Verification items for the finished model (mm, model axes). Face numbers are marked on the shaded views. A direction names the side the tool comes from. Round coordinates to 2 decimals unless told otherwise and drop trailing zeros. Order: outer loops, then holes, each group sorted by start corner. A loop starts at its lowest first (then second) coordinate and runs counter-clockwise, first axis right, second up. Notation, with made-up numbers: (5, 75.5) -> (64, 75.5) arc R13 ccw to (64, 100.5) -> close; hole circle Ø7 at (63, 32.25). An arc over 180 degrees is marked (long way). Return JSON: item names as keys, results as strings. Group by question number.
1) Scan lines: L1, parallel to Y at x = 4, z = 4.5; L2, parallel to Y at x = 76, z = 0.9; L3, parallel to X at y = 53, z = 9.5. Record each from-to range of solid material in increasing order.
2) Section check C-C on x = 18. Enter the section's corners in (y, z), plus the area to 3 significant figures.
3) Section check A-A on x = 40. Enter the section's corners in (y, z).
4) Draft check along X on the marked faces 1, 2 and 3. Enter one of: pulls with the +X half, pulls with the -X half, needs draft (parallel to the pull), parting line crosses it, or undercut.
5) Section check D-D on y = 42. Enter the section's corners in (x, z), plus the area to 3 significant figures.
6) Depth check by flat-ended pin: pin 1 (2.5 mm diameter, centred on y = 85, z = 14, fed in from -X); pin 2 (5 mm diameter, centred on y = 46.5, z = 10, fed in from -X); pin 3 (8 mm diameter, centred on x = 19, z = 9, fed in from +Y). Enter the tip coordinate at first touch or a pass-through.
7) Section check B-B on z = 27.5. Enter the section's corners in (x, y).
8) Tool access check on the marked faces 4, 5, 6 and 7. Record the directions out of +Z, -Z, +X, -X, +Y, -Y that give a thin tool (end or side, any length) a straight path to the whole face; none if there is none.
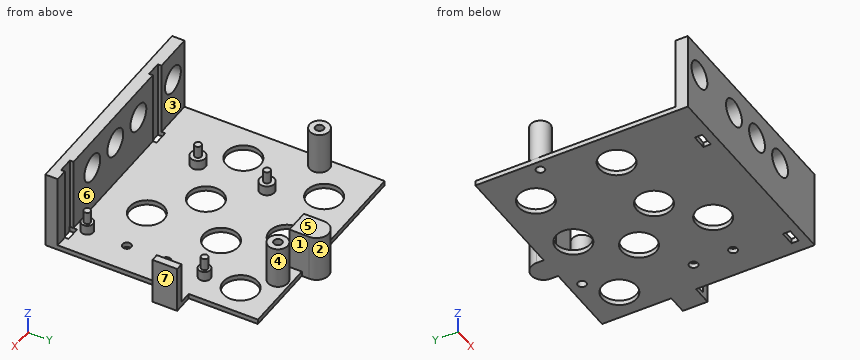
```python
from build123d import *

# Parameters (mm, degrees)
PAD_DEPTH       = 2
SKETCH003_R     = 1.75
SKETCH003_R_2   = 7
SKETCH003_W     = 6
SKETCH003_H     = 3
POCKET_DEPTH    = 5
SKETCH001_R     = 4
SKETCH001_W     = 3
SKETCH001_H     = 10
PAD001_DEPTH    = 17
SKETCH007_R     = 2.4
SKETCH007_R_2   = 3
PAD002_DEPTH    = 4
PAD003_DEPTH    = 30
SKETCH008_R     = 1.35
PAD004_DEPTH    = 5
SKETCH004_R     = 1.7
POCKET001_DEPTH = 19
SKETCH006_R     = 5.5
POCKET002_DEPTH = 5


with BuildPart() as part:
    # Sketch → Pad (new body)
    with BuildSketch(Plane.XY):
        with BuildLine():
            Line((0, 0), (0, 86))
            Line((0, 86), (47.5, 86))
            Line((47.5, 86), (47.5, 89))
            ThreePointArc((57.5, 89), (52.5, 94), (47.5, 89))
            Line((57.5, 89), (57.5, 86))
            Line((57.5, 86), (88, 86))
            Line((88, 58), (88, 86))
            Line((96, 58), (88, 58))
            Line((96, 48), (96, 58))
            Line((88, 48), (96, 48))
            Line((88, 0), (88, 48))
            Line((88, 0), (0, 0))
        make_face()
    extrude(amount=PAD_DEPTH)

    # Sketch003 → Pocket (cut)
    with BuildSketch(Plane.XY.offset(2)):
        with Locations((76, 42)):
            Circle(SKETCH003_R)
        with Locations((76, 26)):
            Circle(SKETCH003_R)
        with Locations((14, 37)):
            Circle(SKETCH003_R_2)
        with Locations((40, 37)):
            Circle(SKETCH003_R_2)
        with Locations((76, 72)):
            Circle(SKETCH003_R_2)
        with Locations((44, 72)):
            Circle(SKETCH003_R_2)
        with Locations((18, 72)):
            Circle(SKETCH003_R_2)
        with Locations((57, 53)):
            Circle(SKETCH003_R_2)
        with Locations((57, 23)):
            Circle(SKETCH003_R_2)
        with Locations((80.1, 5)):
            Rectangle(SKETCH003_W, SKETCH003_H)
        with Locations((18.9, 5)):
            Rectangle(SKETCH003_W, SKETCH003_H)
    extrude(amount=-POCKET_DEPTH, mode=Mode.SUBTRACT)

    # Sketch001 → Pad001 (new body)
    with BuildSketch(Plane.XY.offset(2)):
        with BuildLine():
            Line((47.5, 89), (47.5, 81))
            Line((47.5, 81), (57.5, 81))
            Line((57.5, 81), (57.5, 89))
            ThreePointArc((57.5, 89), (52.5, 94), (47.5, 89))
        make_face()
        with Locations((4, 62)):
            Circle(SKETCH001_R)
        with Locations((94.5, 53)):
            Rectangle(SKETCH001_W, SKETCH001_H)
        with Locations((65.5, 81)):
            Circle(SKETCH001_R)
    extrude(amount=PAD001_DEPTH)

    # Sketch007 → Pad002 (new body)
    with BuildSketch(Plane.XY.offset(2)):
        with Locations((77, 58)):
            Circle(SKETCH007_R)
        with Locations((24.9, 52.9)):
            Circle(SKETCH007_R_2)
        with Locations((24.9, 25)):
            Circle(SKETCH007_R_2)
        with Locations((75.7, 9.8)):
            Circle(SKETCH007_R)
    extrude(amount=PAD002_DEPTH)

    # Sketch005 → Pad003 (new body)
    with BuildSketch(Plane.XY.offset(2)):
        Polygon((0, 0), (0, 5), (15.9, 5), (15.9, 3.5), (22, 3.5), (22, 5), (77, 5), (77, 3.5), (83.1, 3.5), (83.1, 5), (88, 5), (88, 0), align=None)
    extrude(amount=PAD003_DEPTH)

    # Sketch008 → Pad004 (new body)
    with BuildSketch(Plane.XY.offset(6)):
        with Locations((24.9, 52.9)):
            Circle(SKETCH008_R)
        with Locations((77, 58)):
            Circle(SKETCH008_R)
        with Locations((24.9, 25)):
            Circle(SKETCH008_R)
        with Locations((75.7, 9.8)):
            Circle(SKETCH008_R)
    extrude(amount=PAD004_DEPTH)

    # Sketch004 → Pocket001 (cut)
    with BuildSketch(Plane.XY.offset(19)):
        with Locations((4, 62)):
            Circle(SKETCH004_R)
        with Locations((65.5, 81)):
            Circle(SKETCH004_R)
    extrude(amount=-POCKET001_DEPTH, mode=Mode.SUBTRACT)

    # Sketch006 → Pocket002 (cut)
    with BuildSketch(Plane.XZ):
        with Locations((8, 20)):
            Circle(SKETCH006_R)
        with Locations((32, 20)):
            Circle(SKETCH006_R)
        with Locations((48, 20)):
            Circle(SKETCH006_R)
        with Locations((64, 20)):
            Circle(SKETCH006_R)
    extrude(amount=-POCKET002_DEPTH, mode=Mode.SUBTRACT)


solid = part.part
```
Check result:
{
 "1": {"L1": "0 to 5, 58 to 60.3, 63.7 to 66", "L2": "0 to 24.25, 27.75 to 40.25, 43.75 to 65, 79 to 86", "L3": "23.55 to 26.25, 93 to 96"},
 "2": {"outline": "(0, 0) -> (3.5, 0) -> (3.5, 32) -> (0, 32) -> close; (6.5, 0) -> (31.26, 0) -> (31.26, 2) -> (6.5, 2) -> close; (42.74, 0) -> (65, 0) -> (65, 2) -> (42.74, 2) -> close; (79, 0) -> (86, 0) -> (86, 2) -> (79, 2) -> close", "area": "220 mm^2"},
 "3": {"outline": "(0, 0) -> (30, 0) -> (30, 2) -> (5, 2) -> (5, 32) -> (0, 32) -> close; (44, 0) -> (66.26, 0) -> (66.26, 2) -> (44, 2) -> close; (77.74, 0) -> (86, 0) -> (86, 2) -> (77.74, 2) -> close"},
 "4": {"face 1": "undercut", "face 2": "parting line crosses it", "face 3": "needs draft"},
 "5": {"outline": "(0, 0) -> (9.1, 0) -> (9.1, 2) -> (0, 2) -> close; (18.9, 0) -> (35.1, 0) -> (35.1, 2) -> (18.9, 2) -> close; (44.9, 0) -> (74.25, 0) -> (74.25, 2) -> (44.9, 2) -> close; (77.75, 0) -> (88, 0) -> (88, 2) -> (77.75, 2) -> close", "area": "130 mm^2"},
 "6": {"pin 1": "x = 47.5", "pin 2": "x = 93", "pin 3": "y = 5"},
 "7": {"outline": "(0, 0) -> (88, 0) -> (88, 5) -> (83.1, 5) -> (83.1, 3.5) -> (77, 3.5) -> (77, 5) -> (22, 5) -> (22, 3.5) -> (15.9, 3.5) -> (15.9, 5) -> (0, 5) -> close"},
 "8": {"face 4": "+Z", "face 5": "+Z, +X, -X, +Y", "face 6": "+Z, +X, -X", "face 7": "+Z, -Z, +X, +Y, -Y"}
}
